Design review of the part built by this model. Coordinates are the model's own, in mm. Give positions to 0.01 mm unless a question says otherwise; leave off trailing zeros. Write each loop counter-clockwise with the first axis right and the second up, starting at its lowest first coordinate (ties: lowest second). Pieces come first, ordered by that corner, then holes. Notation, with made-up numbers: (80.5, 64) -> (127.5, 64) arc R21 ccw to (127.5, 90) -> close; hole circle Ø6 at (11.25, -27). An arc over 180 degrees is marked (long way). Put each result on its own line as item: value. Start each with the question number.
from build123d import *

# Parameters (mm, degrees)
SKETCH1_R                 = 14.5
BOSS_EXTRUDE1_DEPTH       = 2
F_2_0MM_DOWEL_HOLE1_D     = 2
F_2_0MM_DOWEL_HOLE1_DEPTH = 42.93
F_2_0MM_DOWEL_HOLE1_TIP   = 0.600860619


with BuildPart() as part:
    # Sketch1 → Boss-Extrude1 (new body)
    with BuildSketch(Plane(origin=(0, 0, 0), x_dir=(1, 0, 0), z_dir=(0, 1, 0))):
        with Locations(Location((0, 0, 0), (0, 0, 270))):
            Circle(SKETCH1_R)
    extrude(amount=BOSS_EXTRUDE1_DEPTH)

    # Ø2.0mm Dowel Hole1
    with Locations(Plane(origin=(0, 2, 0), x_dir=(1, 0, 0), z_dir=(0, 1, 0))):
        with Locations((-10, 0), (0, 10), (10, 0), (0, -10)):
            Hole(F_2_0MM_DOWEL_HOLE1_D / 2, depth=F_2_0MM_DOWEL_HOLE1_DEPTH)
            with Locations((0, 0, -(F_2_0MM_DOWEL_HOLE1_DEPTH + F_2_0MM_DOWEL_HOLE1_TIP / 2))):  # 118° drill point
                Cone(0, F_2_0MM_DOWEL_HOLE1_D / 2, F_2_0MM_DOWEL_HOLE1_TIP, mode=Mode.SUBTRACT)


solid = part.part
Q1. Take a section at D-D on z = 0. Give the boundary of the cut face in (x, y).
Q2. Take a section at B-B on z = 10. Give the boundary of the cut face in (x, y).
Q3. Mouldability with a two-part tool opening along Z and no side actions: class faces 1 (the face through (-5.554, 0.986, 13.394)), 2 (the face through (0, 1, 9)), 3 (the face through (0, 2, 0)) as +Z half, -Z half, draft (parallel to the pull), parting line (faces both ways), or undercut.
Q4. Take a section at A-A on x = -10. Give the boundary of the cut face in (y, z), then the cut area to 3 significant figures.
Q5. For pin 1 (1 mm diameter, centred on x = -4, y = 0.5, fed in from -Z), flat-tipped, find the tip position at first contact; note if it passes through.
Q6. To check wall thickness, follow probe 1 along X at (y, z) = (1.6, -9.5); probe 2 along X at (y, z) = (1.5, -10.25); probe 3 along Z at (x, y) = (-10, 1.25). State the ranges of each line that lie inside material, in increasing order. Write a range as from..to.
Q7. Take a section at C-C on x = 0. Give the boundary of the cut face in (y, z).
Result:
1. outline: (-14.5, 0) -> (-11, 0) -> (-11, 2) -> (-14.5, 2) -> close; (-9, 0) -> (9, 0) -> (9, 2) -> (-9, 2) -> close; (11, 0) -> (14.5, 0) -> (14.5, 2) -> (11, 2) -> close
2. outline: (-10.5, 0) -> (-1, 0) -> (-1, 2) -> (-10.5, 2) -> close; (1, 0) -> (10.5, 0) -> (10.5, 2) -> (1, 2) -> close
3. face 1: parting line
3. face 2: undercut
3. face 3: draft
4. outline: (0, -10.5) -> (2, -10.5) -> (2, -1) -> (0, -1) -> close; (0, 1) -> (2, 1) -> (2, 10.5) -> (0, 10.5) -> close
4. area: 38.0 mm^2
5. pin 1: stops at z = -14.07
6. probe 1: x = -10.95..-0.87, 0.87..10.95
6. probe 2: x = -10.26..-0.97, 0.97..10.26
6. probe 3: z = -10.5..-1, 1..10.5
7. outline: (0, -14.5) -> (2, -14.5) -> (2, -11) -> (0, -11) -> close; (0, -9) -> (2, -9) -> (2, 9) -> (0, 9) -> close; (0, 11) -> (2, 11) -> (2, 14.5) -> (0, 14.5) -> close
